Could you check a few things on this model? Use its own coordinates, in mm. A direction names the side the tool comes from. Coordinates: 2 decimals unless noted, no trailing zeros. Loops run counter-clockwise (first coordinate to the right, second up) from the corner with the lowest first, then second, coordinate; pieces in that order, holes last. Notation, with made-up numbers: (-20, 88) -> (2, 88) arc R21 cw to (2, 102) -> close; hole circle Ø3 at (7, 45.5). An arc over 180 degrees is marked (long way). One line per question, with ' | ' between items.
```python
from build123d import *

# Parameters (mm, degrees)
BOSS_EXTRUDE1_REACH             = 42
SKETCH2_W                       = 16
SKETCH2_H                       = 16
SKETCH2_W_2                     = 12
SKETCH2_H_2                     = 12
BOSS_EXTRUDE1_DIRECTION_2_DEPTH = 4
SKETCH3_W                       = 12
SKETCH3_H                       = 12
CUT_EXTRUDE1_DEPTH              = 10
SKETCH4_R                       = 1.7
CUT_EXTRUDE2_DEPTH              = 3
SKETCH5_R                       = 1.7
CUT_EXTRUDE3_DEPTH              = 3
SKETCH6_R                       = 3
CUT_EXTRUDE4_DEPTH              = 13
CUT_EXTRUDE4_DEPTH_BACK         = 1
SKETCH7_R                       = 3
CUT_EXTRUDE5_DEPTH              = 13
CUT_EXTRUDE5_DEPTH_BACK         = 1


with BuildPart() as part:
    # Sketch1 → Revolve1 (revolve)
    with BuildSketch(Plane.XY):
        with BuildLine():
            Line((0, 0), (0, 40))
            ThreePointArc((0, 40), (20, 20), (0, 0))
        make_face()
    revolve(axis=Axis((0, 0, 0), (0, 1, 0)))

    # Sketch2 → Boss-Extrude1 (add, up to next)
    with BuildSketch(Plane(origin=(0, 0, 0), x_dir=(1, 0, 0), z_dir=(0, 1, 0)), mode=Mode.PRIVATE) as boss_extrude1_sk1:
        Rectangle(SKETCH2_W, SKETCH2_H)
        Rectangle(SKETCH2_W_2, SKETCH2_H_2, mode=Mode.SUBTRACT)
    boss_extrude1_tool1 = extrude(boss_extrude1_sk1.sketch, amount=BOSS_EXTRUDE1_REACH, mode=Mode.PRIVATE) - part.part
    add(boss_extrude1_tool1.solids().sort_by_distance((0, 0, -7.773726))[0])

    # Sketch2 → Boss-Extrude1 direction 2 (add)
    with BuildSketch(Plane(origin=(0, 0, 0), x_dir=(1, 0, 0), z_dir=(0, 1, 0))):
        Rectangle(SKETCH2_W, SKETCH2_H)
        Rectangle(SKETCH2_W_2, SKETCH2_H_2, mode=Mode.SUBTRACT)
    extrude(amount=-BOSS_EXTRUDE1_DIRECTION_2_DEPTH)

    # Sketch3 → Cut-Extrude1 (cut)
    with BuildSketch(Plane.XZ.offset(4)):
        Rectangle(SKETCH3_W, SKETCH3_H)
    extrude(amount=-CUT_EXTRUDE1_DEPTH, mode=Mode.SUBTRACT)

    # Sketch4 → Cut-Extrude2 (cut)
    with BuildSketch(Plane(origin=(0, 0, 6), x_dir=(-1, 0, 0), z_dir=(0, 0, -1))):
        with Locations((3, 0)):
            Circle(SKETCH4_R)
    extrude(amount=-CUT_EXTRUDE2_DEPTH, mode=Mode.SUBTRACT)

    # Sketch5 → Cut-Extrude3 (cut)
    with BuildSketch(Plane.XY.offset(-6)):
        with Locations((3, 0)):
            Circle(SKETCH5_R)
    extrude(amount=-CUT_EXTRUDE3_DEPTH, mode=Mode.SUBTRACT)

    # Sketch6 → Cut-Extrude4 (cut, two sides)
    with BuildSketch(Plane(origin=(0, 0, -8), x_dir=(-1, 0, 0), z_dir=(0, 0, -1))) as cut_extrude4_sk:
        with Locations((-3, 0)):
            Circle(SKETCH6_R)
    extrude(amount=CUT_EXTRUDE4_DEPTH, mode=Mode.SUBTRACT)
    extrude(cut_extrude4_sk.sketch, amount=-CUT_EXTRUDE4_DEPTH_BACK, mode=Mode.SUBTRACT)

    # Sketch7 → Cut-Extrude5 (cut, two sides)
    with BuildSketch(Plane.XY.offset(8)) as cut_extrude5_sk:
        with Locations((-3, 0)):
            Circle(SKETCH7_R)
    extrude(amount=CUT_EXTRUDE5_DEPTH, mode=Mode.SUBTRACT)
    extrude(cut_extrude5_sk.sketch, amount=-CUT_EXTRUDE5_DEPTH_BACK, mode=Mode.SUBTRACT)


solid = part.part
```
Q1. Imagine slicing it at B-B on x = -3. Write out the boundary of the cut face in (y, z), plus the area to 3 significant figures.
Values follow:
outline: (-4, -8) -> (1.92, -8) arc R19.77 ccw (long way) to (3, 10.1) -> (3, 7) -> (1.7, 7) -> (1.7, 6) -> (6, 6) -> (6, -6) -> (-4, -6) -> close; (-4, 6) -> (-1.7, 6) -> (-1.7, 7) -> (-3, 7) -> (-3, 8) -> (-4, 8) -> close | area: 1,170 mm2
Q2. Imagine slicing it at C-C on z = 5. Write out the boundary of the cut face in (x, y), plus the area to 3 significant figures.
Values follow:
outline: (-8, -4) -> (-6, -4) -> (-6, 6) -> (6, 6) -> (6, -4) -> (8, -4) -> (8, 2.36) arc R19.36 ccw (long way) to (-8, 2.36) -> close | area: 1,140 mm2
Q3. We'd pull the mould along Z, two halves only. Please class faces 1 (the face through (-3, -2, 7)), 2 (the face through (7, -4, 0)), 3 (the face through (0, 1, 6)): released by +Z, released by -Z, zero draft, split by the parting line, or undercut.
Values follow:
face 1: released by +Z | face 2: zero draft | face 3: undercut
Q4. For faces 4 (the face through (-3, 3, 8)), 5 (the face through (0, 6, 0)), 6 (the face through (4.62, 0.51, -6.49)), which set-ups out of +Z, -Z, +X, -X, +Y, -Y let a thin tool reach every point of the face, with its end or its side?
Values follow:
face 4: +Z | face 5: -Y | face 6: -Z
Q5. Please list where these lines run through material, in increasing order: L1, parallel to Y at x = 3, z = -6.35; L2, parallel to Z at x = -5.5, y = 3; L3, parallel to Z at x = 7, y = 25.5. Write a range as [from, to].
Values follow:
L1: y = [-4, -1.7], [1.7, 38.73] | L2: z = [-8.99, -6], [6, 8.99] | L3: z = [-17.91, 17.91]
Q6. Imagine slicing it at D-D on y = 32. Write out the boundary of the cut face in (x, z).
Values follow:
outline: circle Ø32 at (0, 0)
Q7. For pin 1 (9.5 mm diameter, centred on x = -2.5, z = -1, fed in from -Y); pin 2 (4 mm diameter, centred on x = -6, y = 4.5, fed in from +Z); pin 3 (1.5 mm diameter, centred on x = 0.5, z = 15, fed in from -Y) (3 decimals); pin 4 (5 mm diameter, centred on y = 0, z = -3, fed in from +X), each with a flat end and sliding along its axis, tell me the tip position at first contact or that it passes through.
Values follow:
pin 1: stops at y = -4 | pin 2: stops at z = 13.65 | pin 3: stops at y = 5.975 | pin 4: stops at x = 9.27
Q8. Imagine slicing it at A-A on y = 0. Write out the boundary of the cut face in (x, z).
Values follow:
outline: (-8, -8) -> (0, -8) -> (0, -7) -> (1.3, -7) -> (1.3, -6) -> (-6, -6) -> (-6, 6) -> (-4.7, 6) -> (-4.7, 7) -> (-6, 7) -> (-6, 8) -> (-8, 8) -> close; (-1.3, 6) -> (6, 6) -> (6, -6) -> (4.7, -6) -> (4.7, -7) -> (6, -7) -> (6, -8) -> (8, -8) -> (8, 8) -> (0, 8) -> (0, 7) -> (-1.3, 7) -> close
